For this review, use the dimensioned drawing (mm, ordinates from the lowest corner) and the shaded views. A direction names the side the tool comes from. Coordinates: 2 decimals unless noted, no trailing zeros. Loops run counter-clockwise (first coordinate to the right, second up) from the corner with the lowest first, then second, coordinate; pieces in that order, holes last. Notation, with made-up numbers: (11, 84) - (63, 84) arc R20 cw to (63, 104) - close; hole circle Ø5 at (6.25, 37.25). An arc over 180 degrees is marked (long way). Use a Markdown table: item, result. Add a question column.
1) Clearance check with a flat-ended pin moving along its axis: pin 1 (1.5 mm diameter, centred on y = 8.5, z = 2, fed in from +X). State where the tip first meets the part, or that it passes through.
2) Add section C-C, the plane x = 56. Give the boundary of the cut face in (y, z).
3) Add section A-A, the plane z = 1. Give the boundary of the cut face in (x, y).
4) To check wall thickness, follow L1, parallel to X at y = 2.75, z = 2.8; L2, parallel to X at y = 6.75, z = 0.3; L3, parallel to Z at x = 50, y = 3.5. State the ranges of each line that lie inside material, in increasing order. Write a range as [from, to].
5) Add section B-B, the plane y = 5.75. Give the boundary of the cut face in (x, z).
6) For the marked faces 1 and 2, list the 3-axis set-ups (+Z, -Z, +X, -X, +Y, -Y) from which the entire face can be reached by the end or side of a thin tool; tool diameter is ignored.
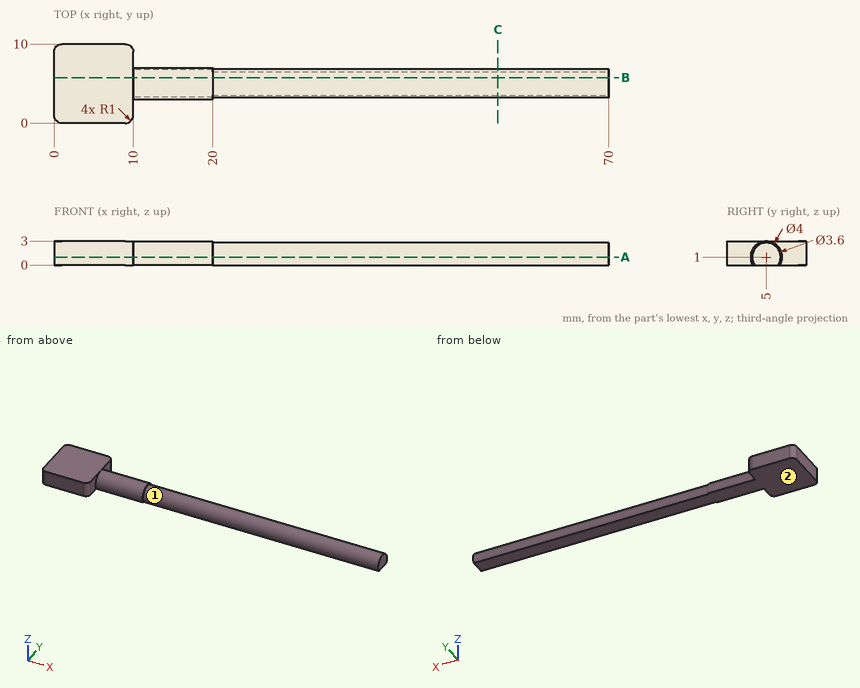
From the geometry:
| question | item | result |
|---|---|---|
| 1 | pin 1 | stops at x = 10 |
| 2 | outline | (3.5, 0) - (6.5, 0) arc R1.8 ccw (long way) to start |
| 3 | outline | (0, 1) arc R1 ccw to (1, 0) - (9, 0) arc R1 ccw to (10, 1) - (10, 3) - (20, 3) - (20, 3.2) - (70, 3.2) - (70, 6.8) - (20, 6.8) - (20, 7) - (10, 7) - (10, 9) arc R1 ccw to (9, 10) - (1, 10) arc R1 ccw to (0, 9) - close |
| 4 | L1 | x = [0, 10] |
| 4 | L2 | x = [0, 20] |
| 4 | L3 | z = [0.01, 1.99] |
| 5 | outline | (0, 0) - (70, 0) - (70, 2.64) - (20, 2.64) - (20, 2.85) - (10, 2.85) - (10, 3) - (0, 3) - close |
| 6 | face 1 | +X |
| 6 | face 2 | -Z, +X, -X, +Y, -Y |
